CAD build for the part. Positions are in the model's coordinates, mm. Coordinates: 2 decimals unless noted, no trailing zeros. Order: outer loops, then holes, each group sorted by start corner. A loop starts at its lowest first (then second) coordinate and runs counter-clockwise, first axis right, second up. Notation, with made-up numbers: (82, 34) - (108, 34) arc R9 ccw to (108, 48) - close; hole circle Ø5 at (-24, 67.5). An arc over 180 degrees is marked (long way). Return JSON: item names as keys, results as strings.
from build123d import *

# Parameters (mm, degrees)
F0_W     = 7
F0_H     = 15
F0_W_2   = 15
F0_H_2   = 5
F0_W_3   = 9
F0_H_3   = 90
F1_DEPTH = 7
F3_R     = 2.6
F4_DEPTH = 16
F5_SIZE  = 6
F6_SIZE  = 6


with BuildPart() as f1:
    # F0 (on Front) → F1 (new body)
    with BuildSketch(Plane.XZ):
        with Locations((0, 7.5)):
            Rectangle(F0_W, F0_H)
        with Locations((-11, 17.5)):
            Rectangle(F0_W_2, F0_H_2)
        with Locations((0, 17.5)):
            Rectangle(F0_W, F0_H_2)
        with Locations((-23, -30)):
            Rectangle(F0_W_3, F0_H_3)
        with Locations((-23, 17.5)):
            Rectangle(F0_W_3, F0_H_2)
    extrude(amount=F1_DEPTH)

    # F2: F1 across plane


with BuildPart() as f1_1:
    add(f1.part)
    add(f1.part.mirror(Plane.YZ))

    # F3 (on Top) → F4 (cut)
    with BuildSketch(Plane.XY):
        with Locations((0, -3.5)):
            Circle(F3_R)
    extrude(amount=F4_DEPTH, mode=Mode.SUBTRACT)

    # F5
    f5_edges = [f1_1.edges().sort_by_distance(p)[0] for p in [
        (-27.5, -7, -27.5),
    ]]
    chamfer(f5_edges, length=F5_SIZE)

    # F6
    f6_edges = [f1_1.edges().sort_by_distance(p)[0] for p in [
        (27.5, 0, -27.5),
    ]]
    chamfer(f6_edges, length=F6_SIZE)


solid = f1_1.part
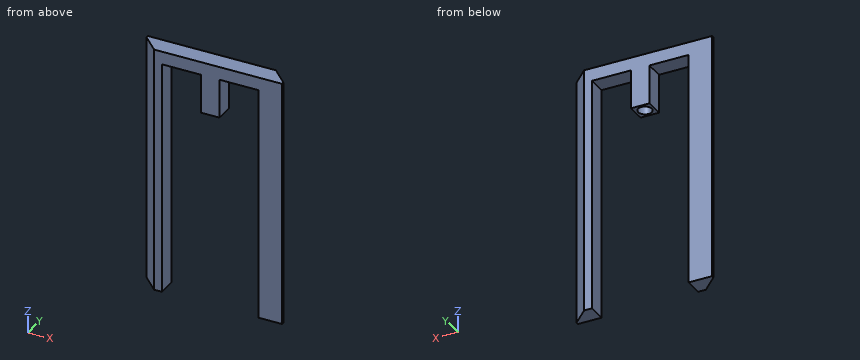
Item 1: Band-saw the part on C-C, the plane x = 0. List the corners of the cut face in (y, z), then the cut area to 3 significant figures.
Findings below:
{"outline": "(-7, 0) - (-6.1, 0) - (-6.1, 16) - (-0.9, 16) - (-0.9, 0) - (0, 0) - (0, 20) - (-7, 20) - close", "area": "56.8 mm²"}
Item 2: Drop flat-ended pins along their axis: P1, Ø2, axis at x = -0.5, y = -3.5, coming from the -Z side; P2, Ø3.5, axis at y = -2.5, z = 6, coming from the +X side; P3, Ø3, axis at x = -1, y = -5.5, coming from the -Z side. Give the stop position or say it passes through.
Findings below:
{"P1": "stops at z = 16", "P2": "stops at x = 25.75", "P3": "stops at z = 0"}
Item 3: Band-saw the part on B-B, the plane z = -6.5. List the corners of the cut face in (x, y).
Findings below:
{"outline": "(-27.5, -1) - (-21.5, -7) - (-18.5, -7) - (-18.5, 0) - (-27.5, 0) - close; (18.5, -7) - (27.5, -7) - (27.5, -6) - (21.5, 0) - (18.5, 0) - close"}
Item 4: Wall check: L1, parallel to Y at x = 0, z = 8.75; L2, parallel to Z at x = -2, y = -3; L3, parallel to X at y = -2.5, z = -4.5. Give the ranges that are in metal, low to high. Write a range as [from, to].
Findings below:
{"L1": "y = [-7, -6.1], [-0.9, 0]", "L2": "z = [16, 20]", "L3": "x = [-26, -18.5], [18.5, 24]"}
Item 5: Band-saw the part on D-D, the plane y = -3.5. List the corners of the cut face in (x, z).
Findings below:
{"outline": "(-25, -75) - (-18.5, -75) - (-18.5, 15) - (-3.5, 15) - (-3.5, 0) - (-2.6, 0) - (-2.6, 16) - (2.6, 16) - (2.6, 0) - (3.5, 0) - (3.5, 15) - (18.5, 15) - (18.5, -75) - (25, -75) - (25, 20) - (-25, 20) - close"}
Item 6: Band-saw the part on A-A, the plane z = 5.5. List the corners of the cut face in (x, y).
Findings below:
{"outline": "(-27.5, -1) - (-21.5, -7) - (-18.5, -7) - (-18.5, 0) - (-27.5, 0) - close; (-3.5, -7) - (3.5, -7) - (3.5, 0) - (-3.5, 0) - close; (18.5, -7) - (27.5, -7) - (27.5, -6) - (21.5, 0) - (18.5, 0) - close; hole circle Ø5.2 at (0, -3.5)"}
